The figure shows three views and two pictorial views of one solid part (mm, origin at its lowest corner). Answer the questions. A direction names the side the tool comes from. Coordinates: 2 decimals unless noted, no trailing zeros. Order: outer loops, then holes, each group sorted by start corner. A loop starts at its lowest first (then second) coordinate and runs counter-clockwise, first axis right, second up.
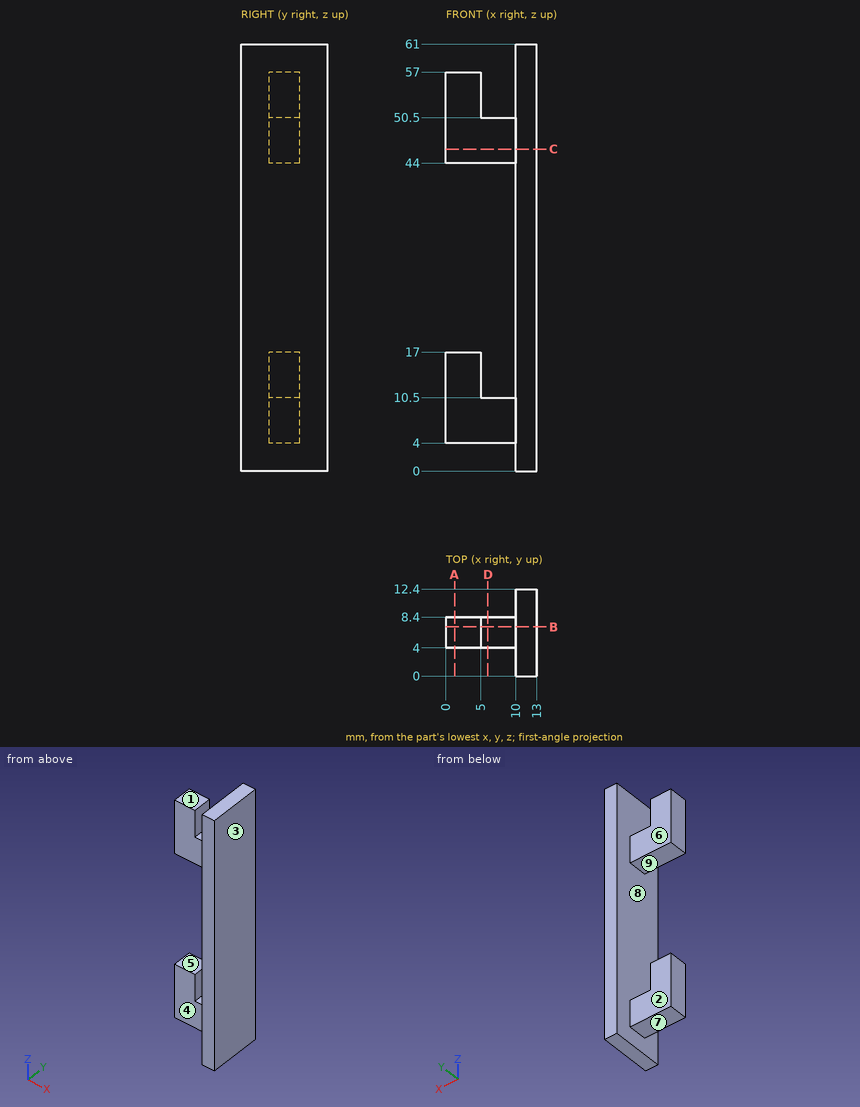
Q1. The part is cut by section C-C, the plane z = 46. Determine the outline of the cut face in (x, y).
Q2. Which of the six approach directions +Z, -Z, +X, -X, +Y, -Y give full straight-line access (tool end or side, diameter ignored) to the marked faces 1, 2, 3, 4 and 5?
Q3. The part is cut by section A-A, the plane x = 1.25. Determine the outline of the cut face in (y, z), then the cut area to 3 significant figures.
Q4. The part is cut by section B-B, the plane y = 7. Determine the outline of the cut face in (x, z), then the cut area to 3 significant figures.
Q5. Determine the mould class of the marked faces 6, 7, 8 and 9 for opening direction Z: +Z half, -Z half, draft (parallel to the pull), parting line (faces both ways), or undercut.
Q6. The part is cut by section D-D, the plane x = 6. Determine the outline of the cut face in (y, z), then the cut area to 3 significant figures.
Q7. Each of these flat-tipped pins is pushed along its axis until it touches: P1, Ø5, axis at x = 5.5, y = 10.5, coming from the -Z side; P2, Ø1.3, axis at x = 2.5, y = 5.5, coming from the +Z side; P3, Ø5, axis at x = 4.5, z = 13.5, coming from the +Y side. Where does it stop, or does it pass through?
Q8. Straight lines are drawn through the part: L1, parallel to X at y = 8, z = 56.5; L2, parallel to Z at x = 9.5, y = 6; L3, parallel to Z at x = 1.75, y = 7.5. For each, find the intervals that lie inside material, in ascending order.
Computed values:
1. outline: (0, 4) - (10, 4) - (10, 0) - (13, 0) - (13, 12.4) - (10, 12.4) - (10, 8.4) - (0, 8.4) - close
2. face 1: +Z, -X, +Y, -Y
2. face 2: +Z, -Z, -X, +Y
2. face 3: +Z, -Z, +X, +Y, -Y
2. face 4: +Z, -Z, -X, -Y
2. face 5: -X, +Y, -Y
3. outline: (4, 4) - (8.4, 4) - (8.4, 17) - (4, 17) - close; (4, 44) - (8.4, 44) - (8.4, 57) - (4, 57) - close
3. area: 114 mm2
4. outline: (0, 4) - (10, 4) - (10, 0) - (13, 0) - (13, 61) - (10, 61) - (10, 50.5) - (5, 50.5) - (5, 57) - (0, 57) - (0, 44) - (10, 44) - (10, 10.5) - (5, 10.5) - (5, 17) - (0, 17) - close
4. area: 378 mm2
5. face 6: draft
5. face 7: -Z half
5. face 8: undercut
5. face 9: undercut
6. outline: (4, 4) - (8.4, 4) - (8.4, 10.5) - (4, 10.5) - close; (4, 44) - (8.4, 44) - (8.4, 50.5) - (4, 50.5) - close
6. area: 57.2 mm2
7. P1: stops at z = 4
7. P2: stops at z = 57
7. P3: stops at y = 8.4
8. L1: x = 0 to 5, 10 to 13
8. L2: z = 4 to 10.5, 44 to 50.5
8. L3: z = 4 to 17, 44 to 57
